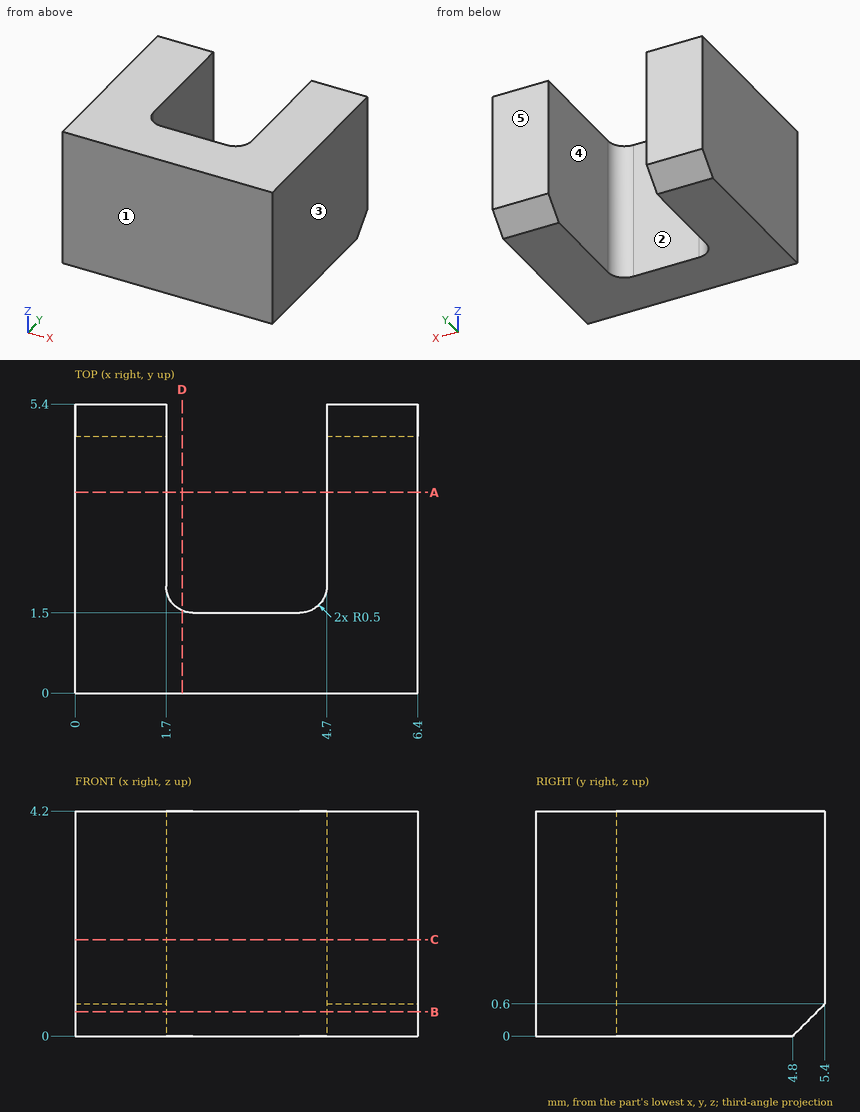
Part print with two shaded views. Sizes in mm from the minimum x, y, z corner. A direction names the side the tool comes from. Round coordinates to 2 decimals unless told otherwise and drop trailing zeros. Loops run counter-clockwise (first coordinate to the right, second up) from the corner with the lowest first, then second, coordinate; pieces in that order, holes last.
1. Slice it at C-C (z = 1.8). Give the cut face in (x, y).
Solutions:
outline: (0, 0) - (6.4, 0) - (6.4, 5.4) - (4.7, 5.4) - (4.7, 2) arc R0.5 cw to (4.2, 1.5) - (2.2, 1.5) arc R0.5 cw to (1.7, 2) - (1.7, 5.4) - (0, 5.4) - close
2. Slice it at B-B (z = 0.45). Give the cut face in (x, y).
Solutions:
outline: (0, 0) - (6.4, 0) - (6.4, 5.25) - (4.7, 5.25) - (4.7, 2) arc R0.5 cw to (4.2, 1.5) - (2.2, 1.5) arc R0.5 cw to (1.7, 2) - (1.7, 5.25) - (0, 5.25) - close
3. Slice it at D-D (x = 2). Give the cut face in (y, z).
Solutions:
outline: (0, 0) - (1.54, 0) - (1.54, 4.2) - (0, 4.2) - close
4. Slice it at A-A (y = 3.75). Give the cut face in (x, z), and give its area (3 significant figures).
Solutions:
outline: (0, 0) - (1.7, 0) - (1.7, 4.2) - (0, 4.2) - close; (4.7, 0) - (6.4, 0) - (6.4, 4.2) - (4.7, 4.2) - close
area: 14.3 mm2
5. Drill centre lines: line 1 along X through (y, z) = (4.9, 1.1); line 2 along Y through (x, z) = (2.25, 3.2); line 3 along Y through (x, z) = (6, 0.3). Where is each one in solid material? Low to high.
Solutions:
line 1: x = 0 to 1.7, 4.7 to 6.4
line 2: y = 0 to 1.5
line 3: y = 0 to 5.1
6. Two-plate mould, pull along X, no slides. Class the marked faces 3, 4 and 5: pulls with the +X half, pulls with the -X half, needs draft (parallel to the pull), parting line crosses it, or undercut.
Solutions:
face 3: pulls with the +X half
face 4: undercut
face 5: needs draft
7. 3-axis set-ups, long thin cutter, end or side, ignore diameter. For the marked faces 1 and 2: which of +Z, -Z, +X, -X, +Y, -Y reach the whole face in a straight line?
Solutions:
face 1: +Z, -Z, +X, -X, -Y
face 2: +Z, -Z, +Y
8. Flat gauge pin, fed straight in: pin 1 (1 mm diameter, centred on x = 3.5, z = 2.5, fed in from +Y). Where does the tip first touch, or does it go through?
Solutions:
pin 1: stops at y = 1.5
